Geometry check sheet. Reference: the model listing, model coordinates, mm. A direction names the side the tool comes from. Round coordinates to 2 decimals unless told otherwise and drop trailing zeros. Write each loop counter-clockwise with the first axis right and the second up, starting at its lowest first coordinate (ties: lowest second). Pieces come first, ordered by that corner, then holes.
Item 1: Scan line: probe 1 along Y at (x, z) = (-5.25, 9.25). Record every from-to range of solid material in increasing order.
Item 2: Depth check by flat-ended pin: P1, Ø1, axis at x = -2, z = 4, coming from the +Y side; P2, Ø4, axis at y = 28, z = 4, coming from the +X side. Enter the tip coordinate at first touch or a pass-through.
Item 3: Cross-section at B-B (x = 4.75). Enter the section's corners in (y, z), then the cut area to 3 significant figures.
Item 4: Access from +Z, -Z, +X, -X, +Y, -Y to the whole of each face (thin tool, end or side, straight path). Record for faces 1 (the face through (-12, 30.4, 0)), 2 (the face through (-8.89, 28, 0)).
Item 5: Cross-section at A-A (z = 2.75). Enter the section's corners in (x, y).
from build123d import *

# Parameters (mm, degrees)
BOSS_EXTRUDE1_DEPTH = 10


with BuildPart() as part:
    # Sketch1 → Boss-Extrude1 (new body, symmetric)
    with BuildSketch(Plane.XY):
        Polygon((-8.89, -25.4), (8.89, -25.4), (8.89, 25.4), (-8.89, 25.4), (-8.89, 30.4), (-15.24, 30.4), (-15.24, -25.4), align=None)
    extrude(amount=BOSS_EXTRUDE1_DEPTH, both=True)


solid = part.part
Resolved:
1. probe 1: y = -25.4 to 25.4
2. P1: stops at y = 25.4
2. P2: stops at x = -8.89
3. outline: (-25.4, -10) - (25.4, -10) - (25.4, 10) - (-25.4, 10) - close
3. area: 1,020 mm2
4. face 1: +Z, -Z, +X, -X, +Y
4. face 2: +Z, -Z, +X, +Y
5. outline: (-15.24, -25.4) - (8.89, -25.4) - (8.89, 25.4) - (-8.89, 25.4) - (-8.89, 30.4) - (-15.24, 30.4) - close
